CAD build for the part. Positions are in the model's coordinates, mm. A direction names the side the tool comes from. Coordinates: 2 decimals unless noted, no trailing zeros. Loops run counter-clockwise (first coordinate to the right, second up) from the corner with the lowest first, then second, coordinate; pieces in that order, holes last. Notation, with made-up numbers: (-6.5, -11) -> (40.5, -11) arc R17 ccw to (40.5, 8) -> close; hole circle Ø10 at (-17.5, 18.5). An arc over 180 degrees is marked (long way). Write item = value, one per line. Start each with the question number.
(1) Band-saw the part on A-A (y = -12). Write the cut outline in (x, z).
(2) Band-saw the part on B-B (x = 0). Write the cut outline in (y, z), and give its area (3 significant figures).
(3) Tool access for faces 1 (the face through (-14, 20, 34)), 2 (the face through (18.16, 21.69, 13.8)), 3 (the face through (22.155, -28.732, 17.255)): list every direction of +Z, -Z, +X, -X, +Y, -Y with a clear straight run to the whole face (end or side of a thin tool).
(4) Flat gauge pin, fed straight in: P1, Ø8, axis at x = -20, y = 20, coming from the +Z side. Where does the tip first touch, or does it go through?
(5) Drill centre lines: line 1 (Y direction, x = -15, z = 31.5); line 2 (Y direction, x = -14.5, z = 32); line 3 (Y direction, x = 5.5, z = 20.5). Where is each one in solid material? Low to high. Write a range as from..to.
(6) Pull direction Y, two halves, no side cores. Call faces 4 (the face through (0, -35, 20)), 5 (the face through (-11, 18, 0)), 6 (the face through (-17.845, -28.732, 17.255)): +Y half, -Y half, draft (parallel to the pull), parting line (faces both ways), or undercut.
(7) Band-saw the part on C-C (z = 15). Count the separate pieces of the cut face and the enclosed holes in it, and give its area (3 significant figures).
```python
from build123d import *

# Parameters (mm, degrees)
F0_W     = 50
F0_H     = 85
F0_R     = 2.5
F0_R_2   = 20
F1_DEPTH = 40
F3_DEPTH = 5
F4_R     = 6
F5_DEPTH = 12


with BuildPart() as f1:
    # F0 (on Top) → F1 (new body)
    with BuildSketch(Plane.XY):
        with Locations((0, 7.5)):
            Rectangle(F0_W, F0_H)
        Polygon((-21.443375673, -27.5), (-18.556624327, -27.5), (-17.1132486541, -30), (-18.556624327, -32.5), (-21.443375673, -32.5), (-22.8867513459, -30), align=None, mode=Mode.SUBTRACT)
        with Locations((-20, -20)):
            Circle(F0_R, mode=Mode.SUBTRACT)
        Polygon((18.556624327, -32.5), (17.1132486541, -30), (18.556624327, -27.5), (21.443375673, -27.5), (22.8867513459, -30), (21.443375673, -32.5), align=None, mode=Mode.SUBTRACT)
        with Locations((20, -20)):
            Circle(F0_R, mode=Mode.SUBTRACT)
        Circle(F0_R_2, mode=Mode.SUBTRACT)
        with Locations((-20, 20)):
            Circle(F0_R, mode=Mode.SUBTRACT)
        Polygon((-18.556624327, 27.5), (-21.443375673, 27.5), (-22.8867513459, 30), (-21.443375673, 32.5), (-18.556624327, 32.5), (-17.1132486541, 30), align=None, mode=Mode.SUBTRACT)
        with Locations((20, 20)):
            Circle(F0_R, mode=Mode.SUBTRACT)
        Polygon((21.443375673, 27.5), (18.556624327, 27.5), (17.1132486541, 30), (18.556624327, 32.5), (21.443375673, 32.5), (22.8867513459, 30), align=None, mode=Mode.SUBTRACT)
    extrude(amount=F1_DEPTH)

    # F2 (on face) → F3 (join)
    with BuildSketch(Plane.XY.offset(40)):
        with BuildLine():
            ThreePointArc((-20, 32.5), (-18.7499999704, 32.1650634924), (-17.8349364564, 31.2499999408))
            Line((-17.8349364564, 31.2499999408), (-18.556624327, 32.5))
            Line((-18.556624327, 32.5), (-20, 32.5))
        make_face()
        with BuildLine():
            ThreePointArc((-22.1650634864, 31.25000004), (-21.24999998, 32.165063521), (-20, 32.5))
            Line((-20, 32.5), (-21.443375673, 32.5))
            Line((-21.443375673, 32.5), (-22.1650634864, 31.25000004))
        make_face()
        with BuildLine():
            ThreePointArc((-22.1650635259, 28.7500000285), (-22.5, 30.0000000396), (-22.1650634864, 31.25000004))
            Line((-22.1650634864, 31.25000004), (-22.8867513459, 30))
            Line((-22.8867513459, 30), (-22.1650635259, 28.7500000285))
        make_face()
        with BuildLine():
            Line((-21.443375673, 27.5), (-20, 27.5))
            ThreePointArc((-20, 27.5), (-21.2500000143, 27.8349364988), (-22.1650635259, 28.7500000285))
            Line((-22.1650635259, 28.7500000285), (-21.443375673, 27.5))
        make_face()
        with BuildLine():
            Line((-18.556624327, 27.5), (-17.8349364673, 28.7500000402))
            ThreePointArc((-17.8349364673, 28.7500000402), (-18.7499999799, 27.8349365022), (-20, 27.5))
            Line((-20, 27.5), (-18.556624327, 27.5))
        make_face()
        with BuildLine():
            ThreePointArc((-17.8349364564, 31.2499999408), (-17.5851854254, 30.6470475798), (-17.5, 30))
            ThreePointArc((-17.5, 30), (-17.5851854283, 29.3529524097), (-17.8349364673, 28.7500000402))
            Line((-17.8349364673, 28.7500000402), (-17.1132486541, 30))
            Line((-17.1132486541, 30), (-17.8349364564, 31.2499999408))
        make_face()
        with BuildLine():
            ThreePointArc((17.8349364866, 31.2499999932), (18.7499999966, 32.1650635075), (20, 32.5))
            Line((20, 32.5), (18.556624327, 32.5))
            Line((18.556624327, 32.5), (17.8349364866, 31.2499999932))
        make_face()
        with BuildLine():
            ThreePointArc((20, 32.5), (21.2499999895, 32.1650635155), (22.1650634973, 31.2500000211))
            Line((22.1650634973, 31.2500000211), (21.443375673, 32.5))
            Line((21.443375673, 32.5), (20, 32.5))
        make_face()
        with BuildLine():
            ThreePointArc((22.1650634973, 31.2500000211), (22.4148145626, 30.6470476245), (22.5, 30))
            ThreePointArc((22.5, 30), (22.41481457, 29.3529524032), (22.1650635259, 28.7500000285))
            Line((22.1650635259, 28.7500000285), (22.8867513459, 30))
            Line((22.8867513459, 30), (22.1650634973, 31.2500000211))
        make_face()
        with BuildLine():
            Line((21.443375673, 27.5), (22.1650635259, 28.7500000285))
            ThreePointArc((22.1650635259, 28.7500000285), (21.2500000143, 27.8349364988), (20, 27.5))
            Line((20, 27.5), (21.443375673, 27.5))
        make_face()
        with BuildLine():
            Line((18.556624327, 27.5), (20, 27.5))
            ThreePointArc((20, 27.5), (18.7499999704, 27.8349365076), (17.8349364564, 28.7500000592))
            Line((17.8349364564, 28.7500000592), (18.556624327, 27.5))
        make_face()
        with BuildLine():
            ThreePointArc((17.8349364564, 28.7500000592), (17.5, 30.0000000302), (17.8349364866, 31.2499999932))
            Line((17.8349364866, 31.2499999932), (17.1132486541, 30))
            Line((17.1132486541, 30), (17.8349364564, 28.7500000592))
        make_face()
        with BuildLine():
            Line((18.556624327, -32.5), (20, -32.5))
            ThreePointArc((20, -32.5), (18.7499999704, -32.1650634924), (17.8349364564, -31.2499999408))
            Line((17.8349364564, -31.2499999408), (18.556624327, -32.5))
        make_face()
        with BuildLine():
            Line((21.443375673, -32.5), (22.1650634973, -31.2500000211))
            ThreePointArc((22.1650634973, -31.2500000211), (21.2499999895, -32.1650635155), (20, -32.5))
            Line((20, -32.5), (21.443375673, -32.5))
        make_face()
        with BuildLine():
            ThreePointArc((22.1650635285, -28.750000033), (22.4148145707, -29.3529524056), (22.5, -30))
            ThreePointArc((22.5, -30), (22.4148145626, -30.6470476245), (22.1650634973, -31.2500000211))
            Line((22.1650634973, -31.2500000211), (22.8867513459, -30))
            Line((22.8867513459, -30), (22.1650635285, -28.750000033))
        make_face()
        with BuildLine():
            ThreePointArc((20, -27.5), (21.2500000165, -27.8349365001), (22.1650635285, -28.750000033))
            Line((22.1650635285, -28.750000033), (21.443375673, -27.5))
            Line((21.443375673, -27.5), (20, -27.5))
        make_face()
        with BuildLine():
            ThreePointArc((17.8349364802, -28.7500000179), (18.7499999911, -27.8349364957), (20, -27.5))
            Line((20, -27.5), (18.556624327, -27.5))
            Line((18.556624327, -27.5), (17.8349364802, -28.7500000179))
        make_face()
        with BuildLine():
            ThreePointArc((17.8349364564, -31.2499999408), (17.5, -29.9999999762), (17.8349364802, -28.7500000179))
            Line((17.8349364802, -28.7500000179), (17.1132486541, -30))
            Line((17.1132486541, -30), (17.8349364564, -31.2499999408))
        make_face()
        with BuildLine():
            Line((-18.556624327, -32.5), (-17.8349364564, -31.2499999408))
            ThreePointArc((-17.8349364564, -31.2499999408), (-18.7499999704, -32.1650634924), (-20, -32.5))
            Line((-20, -32.5), (-18.556624327, -32.5))
        make_face()
        with BuildLine():
            Line((-21.443375673, -32.5), (-20, -32.5))
            ThreePointArc((-20, -32.5), (-21.2499999493, -32.1650635387), (-22.165063451, -31.2500001013))
            Line((-22.165063451, -31.2500001013), (-21.443375673, -32.5))
        make_face()
        with BuildLine():
            ThreePointArc((-22.165063451, -31.2500001013), (-22.5, -30.000000064), (-22.165063515, -28.7500000096))
            Line((-22.165063515, -28.7500000096), (-22.8867513459, -30))
            Line((-22.8867513459, -30), (-22.165063451, -31.2500001013))
        make_face()
        with BuildLine():
            ThreePointArc((-22.165063515, -28.7500000096), (-21.2500000048, -27.8349364933), (-20, -27.5))
            Line((-20, -27.5), (-21.443375673, -27.5))
            Line((-21.443375673, -27.5), (-22.165063515, -28.7500000096))
        make_face()
        with BuildLine():
            ThreePointArc((-20, -27.5), (-18.7499999704, -27.8349365076), (-17.8349364564, -28.7500000592))
            Line((-17.8349364564, -28.7500000592), (-18.556624327, -27.5))
            Line((-18.556624327, -27.5), (-20, -27.5))
        make_face()
        with BuildLine():
            ThreePointArc((-17.8349364564, -28.7500000592), (-17.5851854254, -29.3529524202), (-17.5, -30))
            ThreePointArc((-17.5, -30), (-17.5851854254, -30.6470475798), (-17.8349364564, -31.2499999408))
            Line((-17.8349364564, -31.2499999408), (-17.1132486541, -30))
            Line((-17.1132486541, -30), (-17.8349364564, -28.7500000592))
        make_face()
    extrude(amount=-F3_DEPTH)

    # F4 (on face) → F5 (cut)
    with BuildSketch(Plane.XY.offset(40)):
        with Locations((-20, -20)):
            Circle(F4_R)
        with Locations((20, -20)):
            Circle(F4_R)
        with Locations((-20, 20)):
            Circle(F4_R)
        with Locations((20, 20)):
            Circle(F4_R)
    extrude(amount=-F5_DEPTH, mode=Mode.SUBTRACT)


solid = f1.part
```
Findings below:
q1.outline = (-25, 0) -> (-16, 0) -> (-16, 40) -> (-25, 40) -> close; (16, 0) -> (25, 0) -> (25, 40) -> (16, 40) -> close
q2.outline = (-35, 0) -> (-20, 0) -> (-20, 40) -> (-35, 40) -> close; (20, 0) -> (50, 0) -> (50, 40) -> (20, 40) -> close
q2.area = 1,800 mm²
q3.face_1 = +Z
q3.face_2 = +Z, -Z
q3.face_3 = -Z
q4.P1 = 28
q5.line_1 = -35..-23.32, -16.68..-13.23, 13.23..16.68, 23.32..50
q5.line_2 = -35..-22.4, -17.6..-13.77, 13.77..17.6, 22.4..50
q5.line_3 = -35..-19.23, 19.23..50
q6.face_4 = -Y half
q6.face_5 = draft
q6.face_6 = undercut
q7.separate_pieces = 1
q7.enclosed_holes = 9
q7.area = 2,830 mm²
